The listing builds one solid part. Answer for the finished solid, in the listing's coordinates (mm). Give positions to 0.01 mm unless a question says otherwise; leave off trailing zeros. Order: outer loops, then holes, each group sorted by start corner. A loop starts at its lowest first (then second) coordinate and runs counter-clockwise, first axis right, second up. Notation, with made-up numbers: M -32.5,20 L 24.5,20 A29 cw 24.5,49 Z; hole C -1.5,74 d6. An arc over 180 degrees is marked long. Answer as a JSON object with one key per item and string values. Group by question number.
```python
from build123d import *

# Parameters (mm, degrees)
SKETCH1_W           = 361.95
SKETCH1_H           = 361.95
BOSS_EXTRUDE1_DEPTH = 3.175
SKETCH2_W           = 76.2
SKETCH2_H           = 3.175
CUT_EXTRUDE1_DEPTH  = 3.175
SKETCH3_R           = 12.0777
SKETCH3_W           = 3.175
SKETCH3_H           = 82.55
SKETCH3_H_2         = 44.45
CUT_EXTRUDE2_DEPTH  = 3.175


with BuildPart() as part:
    # Sketch1 → Boss-Extrude1 (new body)
    with BuildSketch(Plane.XY):
        Rectangle(SKETCH1_W, SKETCH1_H)
    extrude(amount=BOSS_EXTRUDE1_DEPTH)

    # Sketch2 → Cut-Extrude1 (cut)
    with BuildSketch(Plane.XY.offset(3.175)):
        with Locations((-60.325, 179.3875)):
            Rectangle(SKETCH2_W, SKETCH2_H)
        with Locations((60.325, 179.3875)):
            Rectangle(SKETCH2_W, SKETCH2_H)
        with Locations((60.325, -179.3875)):
            Rectangle(SKETCH2_W, SKETCH2_H)
        with Locations((-60.325, -179.3875)):
            Rectangle(SKETCH2_W, SKETCH2_H)
    extrude(amount=-CUT_EXTRUDE1_DEPTH, mode=Mode.SUBTRACT)

    # Sketch3 → Cut-Extrude2 (cut)
    with BuildSketch(Plane.XY.offset(3.175)):
        with Locations((0, 90.4875)):
            Circle(SKETCH3_R)
        with Locations((86.058726518, 27.962175279)):
            Circle(SKETCH3_R)
        with Locations((53.187218017, -73.205925279)):
            Circle(SKETCH3_R)
        with Locations((-53.187218017, -73.205925279)):
            Circle(SKETCH3_R)
        with Locations((-86.058726518, 27.962175279)):
            Circle(SKETCH3_R)
        with Locations((-179.3875, 139.7)):
            Rectangle(SKETCH3_W, SKETCH3_H)
        with Locations((-179.3875, 0)):
            Rectangle(SKETCH3_W, SKETCH3_H_2)
        with Locations((-179.3875, -139.7)):
            Rectangle(SKETCH3_W, SKETCH3_H)
        with Locations((179.3875, -139.7)):
            Rectangle(SKETCH3_W, SKETCH3_H)
        with Locations((179.3875, 0)):
            Rectangle(SKETCH3_W, SKETCH3_H_2)
        with Locations((179.3875, 139.7)):
            Rectangle(SKETCH3_W, SKETCH3_H)
    extrude(amount=-CUT_EXTRUDE2_DEPTH, mode=Mode.SUBTRACT)


solid = part.part
```
Item 1: Section C-C (z = 0.5) is taken. Count the separate pieces of the cut face and the enclosed holes in it, and give its area (3 significant figures).
Item 2: Determine the mould class of faces 1 (the cylindrical face through (-87.631, 39.937, 1.61)), 2 (the flat face through (-3, 3, 3.175)) for opening direction X: released by +X, released by -X, zero draft, split by the parting line, or undercut.
Item 3: Section D-D (y = 3) is taken. Determine the outline of the cut face in (x, z) (3 decimals), and give its area (3 significant figures).
Item 4: Flat-ended cylindrical pins translate along their axes: P1, Ø1.6, axis at x = -75, z = 2, coming from the +Y side; P2, Ø1.6, axis at y = -180, z = 2, coming from the -X side; P3, Ø1.6, axis at y = -159.5, z = 1, coming from the +X side. Find the tip coordinate at first contact, or state that the pin passes through.
Item 5: Section B-B (x = -94) is taken. Determine the outline of the cut face in (y, z) (3 decimals), and give its area (3 significant figures).
Item 6: Consider probe 1 along X at (y, z) = (-81, 2.3) (3 decimals); probe 2 along X at (y, z) = (32, 1.65) (3 decimals); probe 3 along Y at (x, z) = (-69.5, 1.2). Determine where each line is inside the solid, lowest interval first. Write a range as from..to.
Item 7: Section A-A (x = 0) is taken. Determine the outline of the cut face in (y, z) (3 decimals).
Values found:
{
 "1": {"separate pieces": "1", "enclosed holes": "5", "area": "126,000 mm^2"},
 "2": {"face 1": "undercut", "face 2": "zero draft"},
 "3": {"outline": "M -177.8,0 L 177.8,0 L 177.8,3.175 L -177.8,3.175 Z", "area": "1,130 mm^2"},
 "4": {"P1": "stops at y = 177.8", "P2": "stops at x = -177.8", "P3": "stops at x = 177.8"},
 "5": {"outline": "M -177.8,0 L 18.862,0 L 18.862,3.175 L -177.8,3.175 Z; M 37.062,0 L 177.8,0 L 177.8,3.175 L 37.062,3.175 Z", "area": "1,070 mm^2"},
 "6": {"probe 1": "x = -180.975..-62.413, -43.961..43.961, 62.413..180.975", "probe 2": "x = -180.975..-97.441, -74.676..74.676, 97.441..180.975", "probe 3": "y = -177.8..177.8"},
 "7": {"outline": "M -180.975,0 L 78.41,0 L 78.41,3.175 L -180.975,3.175 Z; M 102.565,0 L 180.975,0 L 180.975,3.175 L 102.565,3.175 Z"}
}
